Geometry: final body of the model. Coordinates: model frame, mm. A direction names the side the tool comes from. Coordinates: 2 decimals unless noted, no trailing zeros. Order: outer loops, then holes, each group sorted by start corner. A loop starts at its lowest first (then second) coordinate and runs counter-clockwise, first axis right, second up. Notation, with made-up numbers: M -11,50.5 L 17,50.5 A30 ccw 17,72.5 Z; hole C 49.5,39.25 d1. An arc over 180 degrees is marked long. Use CSV: the item, a comma, the result in double quotes. Start each with the question number.
1. Pull-direction query (Z, two-part tool) for faces 4 (the flat face through (0, 0, 45.594)), 5 (the cylindrical face through (-0.33, 2.52, 41.21)), 6 (the flat face through (-0.2, -6.5, 10.188)); classes: pulls with the +Z half, pulls with the -Z half, needs draft (parallel to the pull), parting line crosses it, or undercut.
2. Set-up query: faces 1 (the flat face through (0, 0, -52.196)), 2 (the flat face through (0.2, -6.5, 3.838)), 3 (the cylindrical face through (-1.93, -8.68, 33.57)). Return all of +Z, -Z, +X, -X, +Y, -Y with unobstructed straight access to the full face (end or side cutting, diameter ignored); none if empty.
3. First-contact query: P1, Ø4, axis at x = -4.5, y = 4.5, coming from the +Z side; P2, Ø12, axis at x = -16.5, z = 8, coming from the +Y side; P3, Ø10, axis at x = 7, z = -13, coming from the -Y side. Flat tips, straight axial feed; report the tip coordinate or a pass-through.
4. Section query A-A on y = 0. Return the cut outline in (x, z), and give its area (3 significant figures).
5. Section query B-B on z = -26.5. Return the cut outline in (x, y), and give its area (3 significant figures).
6. Section query C-C on y = 12. State how many separate pieces and enclosed holes the cut face has, and give its area (3 significant figures).
7. Material intervals for line 1 (Z direction, x = -6.5, y = -5); line 2 (Y direction, x = -0.5, z = 3.5); line 3 (X direction, y = 5.5, z = -39), sorted ascending.
from build123d import *


with BuildPart() as f1:
    # F0 (on Front) → F1 (revolve)
    with BuildSketch(Plane.XZ):
        Polygon((0, 36.704396), (0, 0), (0, -52.195604), (25.4, -52.195604), (10.048355, -27.912087), (15.072527, -27.912087), (15.072527, -21.562087), (6.35, -21.562087), (6.35, 3.837913), (15.072527, 3.837913), (15.072527, 10.187913), (6.35, 10.187913), (6.35, 30.354396), (8.89, 30.354396), (8.89, 36.704396), (6.35, 36.704396), (2.54, 36.704396), (2.54, 45.594396), (0, 45.594396), align=None)
    revolve(axis=Axis((0, 0, 18.352198), (0, 0, 1)))


solid = f1.part
Results list:
1,face 4,"pulls with the +Z half"
1,face 5,"needs draft"
1,face 6,"undercut"
2,face 1,"-Z, +X, -X, +Y, -Y"
2,face 2,"none"
2,face 3,"+Z"
3,P1,"stops at z = 36.7"
3,P2,"stops at y = 10.81"
3,P3,"stops at y = -6.03"
4,outline,"M -25.4,-52.2 L 25.4,-52.2 L 10.05,-27.91 L 15.07,-27.91 L 15.07,-21.56 L 6.35,-21.56 L 6.35,3.84 L 15.07,3.84 L 15.07,10.19 L 6.35,10.19 L 6.35,30.35 L 8.89,30.35 L 8.89,36.7 L 2.54,36.7 L 2.54,45.59 L -2.54,45.59 L -2.54,36.7 L -8.89,36.7 L -8.89,30.35 L -6.35,30.35 L -6.35,10.19 L -15.07,10.19 L -15.07,3.84 L -6.35,3.84 L -6.35,-21.56 L -15.07,-21.56 L -15.07,-27.91 L -10.05,-27.91 Z"
4,area,"1,980 mm²"
5,outline,"C 0,0 d30.15"
5,area,"714 mm²"
6,separate pieces,"3"
6,enclosed holes,"0"
6,area,"816 mm²"
7,line 1,"z = -52.2 to -21.56, 3.84 to 10.19, 30.35 to 36.7"
7,line 2,"y = -6.33 to 6.33"
7,line 3,"x = -16.15 to 16.15"
